Geometry: final body of the model. Coordinates: model frame, mm. A direction names the side the tool comes from. Round coordinates to 2 decimals unless told otherwise and drop trailing zeros. Loops run counter-clockwise (first coordinate to the right, second up) from the corner with the lowest first, then second, coordinate; pieces in that order, holes last. Notation, with made-up numbers: M 88.5,87 L 137.5,87 A11 cw 137.5,104 Z; hole C 48.25,-21 d3. An arc over 180 degrees is marked long. Write each question's results on one line, items separated by ' | '.
Autodesk Inventor part; units mm, degrees
ref_plane "Płaszczyzna początkowa" through (0, 0, 0) normal (1, 0, 0) x (0, 1, 0)
ref_plane "XZ Plane" through (0, 0, 0) normal (0, 1, 0) x (-1, 0, 0)
ref_plane "XY Plane" through (0, 0, 0) normal (0, 0, 1) x (1, 0, 0)
sketch "Szkic główny" plane through (0, 0, 0) normal (0, 0, 1) x (1, 0, 0)
  line L0 (0, 0) -> (150, 0)
  line L1 (0, 0) -> (0, 12.5)
  line L2 (150, 12.5) -> (150, 0)
  line L3 (0, 12.5) -> (150, 12.5)
  dimension "d3" = 25
revolve "Obrót1" add sketch "Szkic główny" angle 360 about axis through (0, 0, 0) along (1, 0, 0)
sketch "Szkic3" plane through (0, 0, 0) normal (-1, 0, 0) x (0, 0, 1)
  point P0 (0, 0)
hole "Otwór1" at (0, 0, 0) direction (1, 0, 0) diameter 4.917 depth 19 tip angle 120
sketch "Szkic4" plane through (150, 0, 0) normal (1, 0, 0) x (0, 0, -1)
  point P0 (0, 0)
hole "Otwór2" at (150, 0, 0) direction (-1, 0, 0) diameter 4.917 depth 18 tip angle 120
equation "\"Length\" = 150"
properties part number "Wał" material "Steel"
1. Draft query along Y for faces 3 (the face through (76.05, 11.923, 3.755)), 4 (the face through (9.633, -0.738, 2.345)), 5 (the face through (0, 0, -3)). Return one class per face: pulls with the +Y half, pulls with the -Y half, needs draft (parallel to the pull), parting line crosses it, or undercut.
Answer key:
face 3: parting line crosses it | face 4: undercut | face 5: needs draft
2. Ray query, probe 1 along Z at (x, y) = (145.5, 0); probe 2 along Z at (x, y) = (89, 0.25); probe 3 along Z at (x, y) = (114.5, 6.75). Return the intervals inside material, ascending.
Answer key:
probe 1: z = -12.5 to -2.46, 2.46 to 12.5 | probe 2: z = -12.5 to 12.5 | probe 3: z = -10.52 to 10.52
3. Section C-C (y = -10). Output: boundary loops of the cut face in (x, z).
Answer key:
outline: M 0,-7.5 L 150,-7.5 L 150,7.5 L 0,7.5 Z
4. Section B-B (z = 7.25). Output: boundary loops of the cut face in (x, y), then the cut area to 3 significant figures.
Answer key:
outline: M 0,-10.18 L 150,-10.18 L 150,10.18 L 0,10.18 Z | area: 3,050 mm²
5. Access query for faces 1 (the face through (150, 0, -3)), 2 (the face through (140.874, -0.738, -2.345)). Directions: +Z, -Z, +X, -X, +Y, -Y. A direction counts if a zero-diameter tool reaches every point of the face in a straight line with its end or side. Return the directions, or none.
Answer key:
face 1: +Z, -Z, +X, +Y, -Y | face 2: +X
6. Section A-A (x = 99.5). Output: boundary loops of the cut face in (y, z), then the cut area to 3 significant figures.
Answer key:
outline: C 0,0 d25 | area: 491 mm²
7. Pin query (flat end, axial travel): P1, Ø1, axis at x = 57.5, y = -0.5, coming from the -Z side; P2, Ø6, axis at x = 109.5, z = 6.5, coming from the +Y side; P3, Ø2, axis at x = 81, y = -3, coming from the +Z side; P4, Ø3, axis at y = 0, z = 0, coming from the +X side. Return the tip coordinate at first contact, or that it passes through.
Answer key:
P1: stops at z = -12.5 | P2: stops at y = 12 | P3: stops at z = 12.34 | P4: stops at x = 131.45
